Autodesk Inventor part; units mm, degrees
ref_plane "YZ Plane" through (0, 0, 0) normal (1, 0, 0) x (0, 1, 0)
ref_plane "XZ Plane" through (0, 0, 0) normal (0, 1, 0) x (-1, 0, 0)
ref_plane "XY Plane" through (0, 0, 0) normal (0, 0, 1) x (1, 0, 0)
sketch "Sketch1" plane through (0, 0, 0) normal (0, 0, 1) x (1, 0, 0)
  line L0 (-150, -15) -> (150, -15)
  line L1 (150, -15) -> (150, 15)
  line L2 (150, 15) -> (-150, 15)
  line L3 (-150, 15) -> (-150, -15)
  line L4 (-150, -15) -> (150, 15) construction
  line L5 (150, -15) -> (-150, 15) construction
  line L6 (-124.5, 20) -> (124.5, 20)
  line L7 (124.5, 20) -> (124.5, 15)
  line L8 (124.5, 15) -> (-124.5, 15)
  line L9 (-124.5, 15) -> (-124.5, 20)
  line L10 (-124.5, 20) -> (124.5, 15) construction
  line L11 (124.5, 20) -> (-124.5, 15) construction
  line L12 (-150, 0) -> (150, 0)
  line L13 (-124.5, -20) -> (124.5, -20)
  line L14 (124.5, -20) -> (124.5, -15)
  line L15 (124.5, -15) -> (-124.5, -15)
  line L16 (-124.5, -15) -> (-124.5, -20)
  line L17 (-124.5, -20) -> (124.5, -15) construction
  line L18 (124.5, -20) -> (-124.5, -15) construction
  point P0 (0, 0)
  point P1 (0, 0)
  point P2 (0, 17.5)
  point P3 (0, 15)
  point P4 (-77.3047, 14.0744)
  point P5 (81.6953, 14.0744)
  point P6 (0, -15)
  point P7 (0, -17.5)
  dimension "d0" = 5
  dimension "d1" = 30
  dimension "d2" = 300
  dimension "d3" = 249
extrude "Plate1" add sketch "Sketch1" along normal blind 5
sketch "Sketch3" plane through (0, 0, 5) normal (0, 0, 1) x (1, 0, 0)
  line L0 (-124.5, -20) -> (124.5, -20)
  line L1 (-7.5, -20) -> (7.5, -20)
  line L2 (7.5, -20) -> (7.5, -5)
  line L3 (7.5, -5) -> (-7.5, -5)
  line L4 (-7.5, -5) -> (-7.5, -20)
  point P0 (0, -5)
  point P1 (0, 0)
  dimension "d19" = 15
extrude "Cut1" cut sketch "Sketch3" against normal blind 5
sketch "Sketch4" plane through (0, 0, 5) normal (0, 0, 1) x (1, 0, 0)
  circle A0 centre (-90, 0) radius 1.6
  circle A1 centre (-90, -10) radius 1.6
  line L0 (-7.5, -5) -> (7.5, -5)
  point P0 (0, 0)
  point P1 (0, -5)
  dimension "d9" = 3.2
  dimension "d10" = 3.2
  dimension "d12" = 10
  dimension "d21" = 90
extrude "Cut2" cut sketch "Sketch4" against normal blind 5
sketch "Sketch5" plane through (0, 0, 5) normal (0, 0, 1) x (1, 0, 0)
  line L0 (-124.5, 20) -> (124.5, 20)
  line L1 (-7.5, 20) -> (7.5, 20)
  line L2 (7.5, 20) -> (7.5, 5)
  line L3 (7.5, 5) -> (-7.5, 5)
  line L4 (-7.5, 5) -> (-7.5, 20)
  line L5 (0, 20) -> (0, 0)
  dimension "d15" = 15
extrude "Cut3" cut sketch "Sketch5" against normal blind 5
sketch "Sketch6" plane through (0, 0, 5) normal (0, 0, 1) x (1, 0, 0)
  line L0 (124.5, -20) -> (7.5, -20)
  line L1 (35, -20) -> (45, -20)
  line L2 (45, -20) -> (45, -15)
  line L3 (45, -15) -> (35, -15)
  line L4 (35, -15) -> (35, -20)
  line L5 (7.5, 5) -> (-7.5, 5)
  line L6 (0, 5) -> (0, -4.2095)
  line L7 (-35, -20) -> (-45, -20)
  line L8 (-45, -20) -> (-45, -15)
  line L9 (-45, -15) -> (-35, -15)
  line L10 (-35, -15) -> (-35, -20)
  point P0 (0, 0)
  dimension "d22" = 5
  dimension "d23" = 10
  dimension "d24" = 35
extrude "Cut4" cut sketch "Sketch6" against normal blind 5
equation "\"d7\" = Thickness"
equation "\"d13\" = Thickness"
equation "\"d16\" = Thickness"
equation "\"d25\" = Thickness"
equation "\"d4\" = Thickness"
equation "\"BendRadius\" = Thickness"
equation "\"BendReliefWidth\" = Thickness"
equation "\"BendReliefDepth\" = 0.5 * Thickness"
equation "\"TransitionRadius\" = BendRadius"
equation "\"JacobiRadiusSize\" = BendRadius"
equation "\"GapSize\" = Thickness"
properties part number "Base Leg V2 Slotted"
Verification items for the finished model (mm, model axes). A direction names the side the tool comes from. Coordinates: 2 decimals unless noted, no trailing zeros. Loops run counter-clockwise (first coordinate to the right, second up) from the corner with the lowest first, then second, coordinate; pieces in that order, holes last. Notation, with made-up numbers: (5, 49.5) -> (19, 49.5) arc R30 ccw to (19, 86.5) -> close; hole circle Ø1 at (-22, 89). An arc over 180 degrees is marked (long way). Answer in a Markdown table with one row per item.
1) Section check D-D (x = 39.5). Record the cut outline in (y, z), and give its area (3 significant figures).
The answers:
| item | result |
|---|---|
| outline | (-15, 0) -> (20, 0) -> (20, 5) -> (-15, 5) -> close |
| area | 175 mm2 |
2) Depth check by flat-ended pin: P1, Ø1.5, axis at y = -17, z = 1.5, coming from the +X side; P2, Ø2.5, axis at x = -3, z = 1.5, coming from the +Y side; P3, Ø1.5, axis at x = -2, z = 1.5, coming from the -Y side. Enter the tip coordinate at first touch or a pass-through.
The answers:
| item | result |
|---|---|
| P1 | stops at x = 124.5 |
| P2 | stops at y = 5 |
| P3 | stops at y = -5 |
3) Section check C-C (x = -128.5). Record the cut outline in (y, z).
The answers:
| item | result |
|---|---|
| outline | (-15, 0) -> (15, 0) -> (15, 5) -> (-15, 5) -> close |
4) Section check B-B (z = 1.4). Give the number of separate pieces and of enclosed holes in the cut face, and give its area (3 significant figures).
The answers:
| item | result |
|---|---|
| separate pieces | 1 |
| enclosed holes | 2 |
| area | 10,900 mm2 |
5) Draft check along X on faces 5 (the face through (35, -17, 3)), 6 (the face through (-124.5, 17, 2)), 7 (the face through (65, 20, 2)). Enter one of: released by +X, released by -X, zero draft, split by the parting line, or undercut.
The answers:
| item | result |
|---|---|
| face 5 | undercut |
| face 6 | released by -X |
| face 7 | zero draft |
6) Section check A-A (y = 7.5). Record the cut outline in (x, z).
The answers:
| item | result |
|---|---|
| outline | (-150, 0) -> (-7.5, 0) -> (-7.5, 5) -> (-150, 5) -> close; (7.5, 0) -> (150, 0) -> (150, 5) -> (7.5, 5) -> close |
7) Access from +Z, -Z, +X, -X, +Y, -Y to the whole of each face (thin tool, end or side, straight path). Record for faces 1 (the face through (124.5, 18, 2)), 2 (the face through (0, 5, 3)), 3 (the face through (-45, -18, 3)), 4 (the face through (-137, 15, 2)).
The answers:
| item | result |
|---|---|
| face 1 | +Z, -Z, +X, +Y |
| face 2 | +Z, -Z, +Y |
| face 3 | +Z, -Z, -Y |
| face 4 | +Z, -Z, -X, +Y |
8) Scan lines: line 1 along X through (y, z) = (-18, 2); line 2 along Y through (x, z) = (-90, 1.75); line 3 along X through (y, z) = (10, 4.6). Record each from-to range of solid material in increasing order. Write a range as from..to.
The answers:
| item | result |
|---|---|
| line 1 | x = -124.5..-45, -35..-7.5, 7.5..35, 45..124.5 |
| line 2 | y = -20..-11.6, -8.4..-1.6, 1.6..20 |
| line 3 | x = -150..-7.5, 7.5..150 |
